The figure shows three views and two pictorial views of one solid part (mm, origin at its lowest corner). Answer the questions. A direction names the side the tool comes from. Coordinates: 2 decimals unless noted, no trailing zeros. Loops run counter-clockwise (first coordinate to the right, second up) from the corner with the lowest first, then second, coordinate; pieces in that order, holes last. Notation, with made-up numbers: M 7,78.5 L 64,78.5 A7 cw 64,84.5 Z; hole C 7.5,-40 d10. An arc over 180 degrees is marked long. Return JSON: item names as keys, results as strings. Group by question number.
1. The mould has two halves that part along Y. Classify the marked faces 1, 2, 3 and 4: pulls with the +Y half, pulls with the -Y half, needs draft (parallel to the pull), parting line crosses it, or undercut.
2. Which of the six approach directions +Z, -Z, +X, -X, +Y, -Y give full straight-line access (tool end or side, diameter ignored) to the marked faces 5, 6, 7 and 8?
3. Straight lines are drawn through the part: L1, parallel to X at y = 7.5, z = 0.1; L2, parallel to X at y = 32, z = 2.9; L3, parallel to X at y = 24, z = 2.45. For each, find the intervals that lie inside material, in ascending order. Write a range as from..to.
4. Section D-D (z = 2.4) is taken. Write down the section's boundary in (x, y), then the cut area to 3 significant figures.
5. Section A-A (y = 25) is taken. Write down the section's boundary in (x, z), then the cut area to 3 significant figures.
6. Given P1, Ø1.5, axis at y = 13.5, z = 1, coming from the -X side, flat-ended and moving along its own axis, determine where the tip first touches the part or whether it passes through.
7. Section B-B (x = 25) is taken. Write down the section's boundary in (y, z).
8. Section C-C (y = 33) is taken. Write down the section's boundary in (x, z), then the cut area to 3 significant figures.
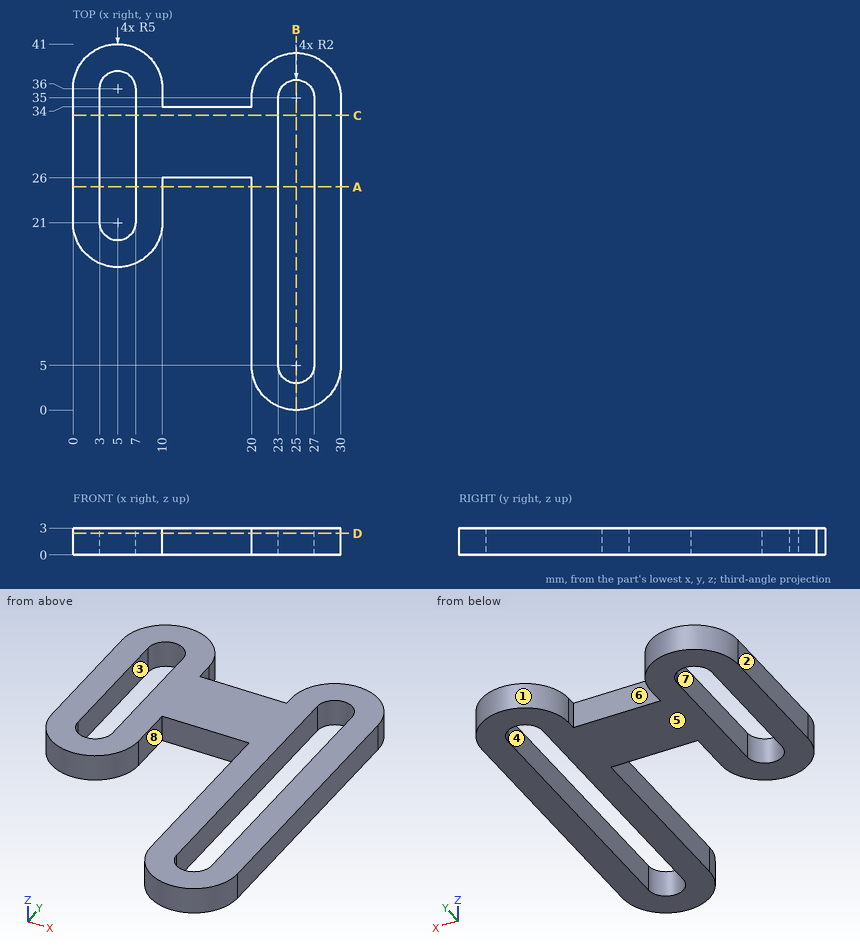
Worked out:
{
 "1": {"face 1": "pulls with the +Y half", "face 2": "needs draft", "face 3": "undercut", "face 4": "undercut"},
 "2": {"face 5": "-Z, +X, -X, +Y, -Y", "face 6": "+Z, -Z, +Y", "face 7": "+Z, -Z", "face 8": "+Z, -Z, -Y"},
 "3": {"L1": "20..23, 27..30", "L2": "0..3, 7..23, 27..30", "L3": "0..3, 7..10, 20..23, 27..30"},
 "4": {"outline": "M 0,21 A5 ccw 10,21 L 10,26 L 20,26 L 20,5 A5 ccw 30,5 L 30,35 A5 ccw 20,35 L 20,34 L 10,34 L 10,36 A5 ccw 0,36 Z; hole M 3,21 A2 ccw 7,21 L 7,36 A2 ccw 3,36 Z; hole M 23,5 A2 ccw 27,5 L 27,35 A2 ccw 23,35 Z", "area": "482 mm^2"},
 "5": {"outline": "M 0,0 L 3,0 L 3,3 L 0,3 Z; M 7,0 L 10,0 L 10,3 L 7,3 Z; M 20,0 L 23,0 L 23,3 L 20,3 Z; M 27,0 L 30,0 L 30,3 L 27,3 Z", "area": "36.0 mm^2"},
 "6": {"P1": "x = 20"},
 "7": {"outline": "M 0,0 L 3,0 L 3,3 L 0,3 Z; M 37,0 L 40,0 L 40,3 L 37,3 Z"},
 "8": {"outline": "M 0,0 L 3,0 L 3,3 L 0,3 Z; M 7,0 L 23,0 L 23,3 L 7,3 Z; M 27,0 L 30,0 L 30,3 L 27,3 Z", "area": "66.0 mm^2"}
}
